Could you check a few things on this model? Use its own coordinates, in mm. A direction names the side the tool comes from. Round coordinates to 2 decimals unless told otherwise and drop trailing zeros. Loops run counter-clockwise (first coordinate to the right, second up) from the corner with the lowest first, then second, coordinate; pieces in that order, holes last. Notation, with made-up numbers: (-12.5, 73) -> (13.5, 73) arc R36 ccw to (13.5, 112) -> close; hole circle Ø2 at (13.25, 31). An arc over 180 degrees is marked (long way). One line per item, written item: value.
```python
from build123d import *

# Parameters (mm, degrees)
SKETCH1_R           = 22.225
SKETCH1_R_2         = 6.35
BOSS_EXTRUDE1_DEPTH = 66.675
SKETCH1_3_W         = 38.1
SKETCH1_3_H         = 38.1
BOSS_EXTRUDE2_DEPTH = 50.8
BOSS_EXTRUDE3_START = -50.8
SKETCH1_4_R         = 6.35
BOSS_EXTRUDE3_DEPTH = 38.1
SKETCH2_R           = 2.38125
CUT_EXTRUDE1_DEPTH  = 12.7
CUT_EXTRUDE2_START  = -25.4
SKETCH2_2_R         = 2.38125
CUT_EXTRUDE2_DEPTH  = 12.7
FILLET1_R           = 3.81


with BuildPart() as part:
    # Sketch1 → Boss-Extrude1 (new body)
    with BuildSketch(Plane(origin=(0, 0, 0), x_dir=(0, 0, -1), z_dir=(1, 0, 0))):
        Circle(SKETCH1_R)
        Circle(SKETCH1_R_2)
        with BuildLine():
            ThreePointArc((11.4476253, 19.05), (0, 22.225), (-11.4476253, 19.05))
            Line((-11.4476253, 19.05), (11.4476253, 19.05))
        make_face()
        with BuildLine():
            Line((19.05, 11.4476253), (19.05, -11.4476253))
            ThreePointArc((19.05, -11.4476253), (21.416545882, -5.939881102), (22.225, 0))
            ThreePointArc((22.225, 0), (21.416545882, 5.939881102), (19.05, 11.4476253))
        make_face()
        with BuildLine():
            Line((11.4476253, -19.05), (-11.4476253, -19.05))
            ThreePointArc((-11.4476253, -19.05), (0, -22.225), (11.4476253, -19.05))
        make_face()
        with BuildLine():
            ThreePointArc((-19.05, 11.4476253), (-22.225, 0), (-19.05, -11.4476253))
            Line((-19.05, -11.4476253), (-19.05, 11.4476253))
        make_face()
    extrude(amount=BOSS_EXTRUDE1_DEPTH)

    # Sketch1<3> → Boss-Extrude2 (add)
    with BuildSketch(Plane(origin=(0, 0, 0), x_dir=(0, 0, -1), z_dir=(1, 0, 0))):
        Rectangle(SKETCH1_3_W, SKETCH1_3_H)
    extrude(amount=-BOSS_EXTRUDE2_DEPTH)

    # Sketch1<4> → Boss-Extrude3 (add)
    with BuildSketch(Plane(origin=(0, 0, 0), x_dir=(0, 0, -1), z_dir=(1, 0, 0)).offset(BOSS_EXTRUDE3_START)):
        Circle(SKETCH1_4_R)
    extrude(amount=-BOSS_EXTRUDE3_DEPTH)

    # Sketch2 → Cut-Extrude1 (cut)
    with BuildSketch(Plane(origin=(0, 19.05, 0), x_dir=(1, 0, 0), z_dir=(0, 1, 0))):
        with Locations(Location((-42.8625, 9.525, 0), (0, 0, 270))):
            Circle(SKETCH2_R)
        with Locations(Location((-7.9375, 9.525, 0), (0, 0, 270))):
            Circle(SKETCH2_R)
        with Locations(Location((-7.9375, -9.525, 0), (0, 0, 90))):
            Circle(SKETCH2_R)
        with Locations(Location((-42.8625, -9.525, 0), (0, 0, 90))):
            Circle(SKETCH2_R)
    extrude(amount=-CUT_EXTRUDE1_DEPTH, mode=Mode.SUBTRACT)

    # Sketch2<2> → Cut-Extrude2 (cut)
    with BuildSketch(Plane(origin=(0, 19.05, 0), x_dir=(1, 0, 0), z_dir=(0, 1, 0)).offset(CUT_EXTRUDE2_START)):
        with Locations(Location((-42.8625, 9.525, 0), (0, 0, 270))):
            Circle(SKETCH2_2_R)
        with Locations(Location((-7.9375, 9.525, 0), (0, 0, 270))):
            Circle(SKETCH2_2_R)
        with Locations(Location((-7.9375, -9.525, 0), (0, 0, 90))):
            Circle(SKETCH2_2_R)
        with Locations(Location((-42.8625, -9.525, 0), (0, 0, 90))):
            Circle(SKETCH2_2_R)
    extrude(amount=-CUT_EXTRUDE2_DEPTH, mode=Mode.SUBTRACT)

    # Fillet1
    fillet1_edges = [part.edges().sort_by_distance(p)[0] for p in [
        (-25.4, 19.05, 19.05),
        (-25.4, 19.05, -19.05),
        (-25.4, -19.05, -19.05),
        (-25.4, -19.05, 19.05),
    ]]
    fillet(fillet1_edges, radius=FILLET1_R)


solid = part.part
```
Item 1: If we section it at B-B on z = 0: List the corners of the cut face in (x, y) for me (3 decimals), plus the area to 3 significant figures.
Output:
outline: (-88.9, -6.35) -> (-50.8, -6.35) -> (-50.8, -19.05) -> (0, -19.05) -> (0, -22.225) -> (66.675, -22.225) -> (66.675, 22.225) -> (0, 22.225) -> (0, 19.05) -> (-50.8, 19.05) -> (-50.8, 6.35) -> (-88.9, 6.35) -> close
area: 5,380 mm²
Item 2: For faces 1 (the face through (-50.8, 5, 5)), 2 (the face through (-7.025, 12.789, 7.325)), 3 (the face through (0, 0, 20)), which set-ups out of +Z, -Z, +X, -X, +Y, -Y let a thin tool reach every point of the face, with its end or its side?
Output:
face 1: -X
face 2: +Y
face 3: +Z, -X, +Y, -Y
Item 3: If we section it at C-C on y = 9: Count the separate pieces of the cut face and the enclosed holes in it, plus the area to 3 significant figures.
Output:
separate pieces: 1
enclosed holes: 4
area: 4,570 mm²
Item 4: Will these pins go through, and if not, where does the flat tip stop? pin 1 Ø1 at (x, y) = (-53.5, -5.5) entering from -Z; pin 2 Ø6 at (x, z) = (-51, 1) entering from -Y; pin 3 Ø3 at (x, z) = (-7.94, 9.52) entering from -Y; pin 4 Ø8 at (x, z) = (-60, 12.5) entering from +Y.
Output:
pin 1: stops at z = -3.91
pin 2: stops at y = -19.05
pin 3: stops at y = -6.35
pin 4: passes through
Item 5: If we section it at A-A on x = -38: List the corners of the cut face in (y, z) for me.
Output:
outline: (-19.05, -15.24) arc R3.81 ccw to (-15.24, -19.05) -> (15.24, -19.05) arc R3.81 ccw to (19.05, -15.24) -> (19.05, 15.24) arc R3.81 ccw to (15.24, 19.05) -> (-15.24, 19.05) arc R3.81 ccw to (-19.05, 15.24) -> close
Item 6: If we mould it in two halves opening along X, with no side actions, what happens to faces 4 (the face through (-43, -6.35, 10)), 5 (the face through (-25.756, 17.904, 17.964)), 6 (the face through (0, -16, -16))? For each: released by +X, released by -X, zero draft, split by the parting line, or undercut.
Output:
face 4: undercut
face 5: zero draft
face 6: released by +X
Item 7: I need wall thicknesses on line 1 (X direction, y = 7, z = -8) (3 decimals); line 2 (X direction, y = 17.5, z = -10) (3 decimals); line 3 (X direction, y = 1.5, z = -10) (3 decimals). Which ranges of each line are inside material? Lowest first, please. Write a range as from..to.
Output:
line 1: x = -50.8..-44.691, -41.034..-9.766, -6.109..66.675
line 2: x = -50.8..-45.196, -40.529..-10.271, -5.604..66.675
line 3: x = -50.8..66.675
